Geometry check sheet. Reference: the model listing, model coordinates, mm. Face numbers are marked on the shaded views. A direction names the side the tool comes from. Round coordinates to 2 decimals unless told otherwise and drop trailing zeros. Loops run counter-clockwise (first coordinate to the right, second up) from the corner with the lowest first, then second, coordinate; pieces in that order, holes last. Notation, with made-up numbers: M -37,-7.5 L 2,-7.5 A17 cw 2,2.5 Z; hole C 61,88 d7. An arc over 180 degrees is marked long. Use one line per item in the form item = value. Start each with the question number.
1. Cross-section at C-C (x = 2.5). Record the boundary of the cut face in (y, z).
2. Cross-section at D-D (y = -2.75). Record the boundary of the cut face in (x, z) (3 decimals), then the cut area to 3 significant figures.
3. Cross-section at B-B (z = 2.8). Record the boundary of the cut face in (x, y) (3 decimals).
4. Material ranges on line 1 (Y direction, x = 0, z = 1.8); line 2 (Z direction, x = -0.25, y = 2.5); line 3 (Y direction, x = 1.5, z = 4.1), recorded low to high.
5. Go/stop test with flat-tipped pins: pin 1 (2 mm diameter, centred on x = 1.5, y = -1.5, fed in from +Z); pin 2 (2 mm diameter, centred on x = 2.5, z = 2, fed in from +Y). Record where each tip stops, or that it passes through.
6. Cross-section at A-A (y = 0). Record the boundary of the cut face in (x, z) (3 decimals), then the cut area to 3 significant figures.
7. Set-up check for the marked faces 1 and 2: record each of +Z, -Z, +X, -X, +Y, -Y from which the full face is reachable in a straight line by a thin tool's end or side.
8. Draft check along Y on the marked faces 3, 4 and 5. Enter one of: pulls with the +Y half, pulls with the -Y half, needs draft (parallel to the pull), parting line crosses it, or undercut.
```python
from build123d import *

# Parameters (mm, degrees)
PAD_DEPTH       = 6
SKETCH001_R     = 2.2
POCKET_DEPTH    = 6.001
POCKET001_DEPTH = 3.5


with BuildPart() as part:
    # Sketch → Pad (new body)
    with BuildSketch(Plane.XY):
        Polygon((-3.525, 6.470319), (-3.525, -6.470319), (0.643078, -6.470319), (5.925, -3.4208), (5.925, 3.4208), (0.643078, 6.470319), align=None)
    extrude(amount=PAD_DEPTH)

    # Sketch001 → Pocket (cut, through all)
    with BuildSketch(Plane.XY.offset(6)):
        Circle(SKETCH001_R)
    extrude(amount=-POCKET_DEPTH, mode=Mode.SUBTRACT)

    # Sketch002 → Pocket001 (cut)
    with BuildSketch(Plane.XY.offset(6)):
        Polygon((0, -4.070319), (3.525, -2.03516), (3.525, 2.03516), (0, 4.070319), (-3.525, 2.03516), (-3.525, -2.03516), align=None)
    extrude(amount=-POCKET001_DEPTH, mode=Mode.SUBTRACT)


solid = part.part
```
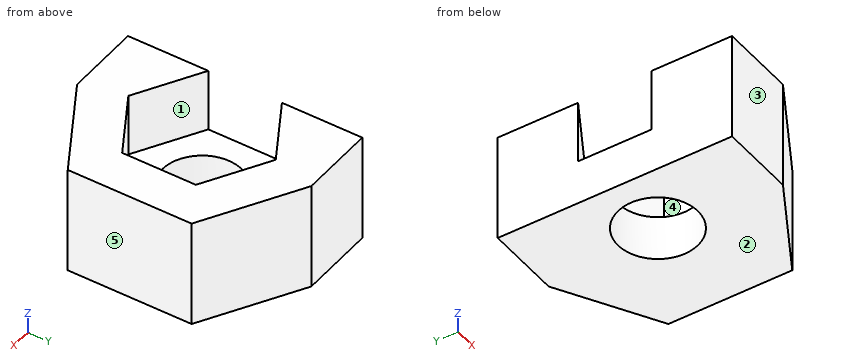
Reported:
q1.outline = M -5.4,0 L 5.4,0 L 5.4,6 L 2.63,6 L 2.63,2.5 L -2.63,2.5 L -2.63,6 L -5.4,6 Z
q2.outline = M -3.525,0 L 5.925,0 L 5.925,6 L 2.287,6 L 2.287,2.5 L -2.287,2.5 L -2.287,6 L -3.525,6 Z
q2.area = 40.7 mm²
q3.outline = M -3.525,-6.47 L 0.643,-6.47 L 5.925,-3.421 L 5.925,3.421 L 0.643,6.47 L -3.525,6.47 L -3.525,2.035 L 0,4.07 L 3.525,2.035 L 3.525,-2.035 L 0,-4.07 L -3.525,-2.035 Z
q4.line_1 = -6.47 to -2.2, 2.2 to 6.47
q4.line_2 = 0 to 2.5
q4.line_3 = -5.98 to -3.2, 3.2 to 5.98
q5.pin_1 = 2.5
q5.pin_2 = 5.98
q6.outline = M -3.525,0 L -2.2,0 L -2.2,2.5 L -3.525,2.5 Z; M 2.2,0 L 5.925,0 L 5.925,6 L 3.525,6 L 3.525,2.5 L 2.2,2.5 Z
q6.area = 21.0 mm²
q7.face_1 = +Z
q7.face_2 = -Z, +X, -X, +Y, -Y
q8.face_3 = pulls with the -Y half
q8.face_4 = undercut
q8.face_5 = needs draft
